Source: CAD feature listing. Evaluate the final solid. Frame: model axes, mm. Face numbers are marked on the shaded views. A direction names the side the tool comes from. Coordinates: 2 decimals unless noted, no trailing zeros. Loops run counter-clockwise (first coordinate to the right, second up) from the corner with the lowest first, then second, coordinate; pieces in that order, holes last. Notation, with made-up numbers: (78.25, 5) -> (101.25, 5) arc R23 ccw to (101.25, 40) -> close; hole circle Ø1 at (-28, 48.5). An arc over 180 degrees is marked (long way). Answer as CSV lines item,"result".
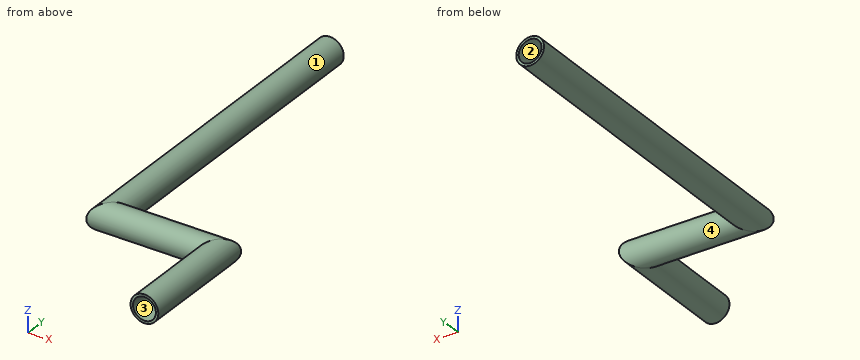
from build123d import *

# Parameters (mm, degrees)
SKETCH2_R   = 12.7
SKETCH2_R_2 = 10.458255758


with BuildPart() as part:
    # Sweep1: sweep along a path in Sketch1
    with BuildLine(Plane.XY) as sweep1_path:
        Line((0, 300), (0, 0))
        Line((0, 0), (99.24397827, 0))
        Line((99.24397827, 0), (99.24397827, -100))
    # Sketch2 → Sweep1 (sweep)
    with BuildSketch(Plane(origin=(0, 300, 0), x_dir=(1, 0, 0), z_dir=(0, 1, 0))):
        Circle(SKETCH2_R)
        Circle(SKETCH2_R_2, mode=Mode.SUBTRACT)
    sweep(path=sweep1_path.line, transition=Transition.RIGHT)


solid = part.part
(1) Cut plane D-D (x = 83). Return the cut outline in (y, z).
Computed values:
outline,"circle Ø25.4 at (0, 0); hole circle Ø20.92 at (0, 0)"
(2) Pin query (flat end, axial travel): pin 1 Ø5 at (x, y) = (4.5, 231) entering from -Z; pin 2 Ø6 at (x, z) = (63.5, 8) entering from -Y; pin 3 Ø12.5 at (x, z) = (0, 0) entering from +Y. Return the tip coordinate at first contact, or that it passes through.
Computed values:
pin 1,"z = -12.54"
pin 2,"y = -11.67"
pin 3,"y = -8.39"
(3) Cut plane B-B (x = 0). Return the cut outline in (y, z), then the cut area to 3 significant figures.
Computed values:
outline,"(0, -12.7) -> (300, -12.7) -> (300, -10.46) -> (0, -10.46) arc R10.46 cw to (0, 10.46) -> (300, 10.46) -> (300, 12.7) -> (0, 12.7) arc R12.7 ccw to start"
area,"1,430 mm^2"
(4) Draft query along Z for the marked faces 1 and 2. Return one class per face: released by +Z, released by -Z, zero draft, split by the parting line, or undercut.
Computed values:
face 1,"split by the parting line"
face 2,"undercut"
(5) Cut plane C-C (y = 0). Return the cut outline in (x, z), then the cut area to 3 significant figures.
Computed values:
outline,"(0, -12.7) -> (99.24, -12.7) arc R12.7 ccw to (99.24, 12.7) -> (0, 12.7) arc R12.7 ccw to start; hole (0, -10.46) -> (99.24, -10.46) arc R10.46 ccw to (99.24, 10.46) -> (0, 10.46) arc R10.46 ccw to start"
area,"608 mm^2"
(6) Material intervals for L1, parallel to X at y = -38, z = 0; L2, parallel to Z at x = 0, y = 233, sorted ascending. Write a range as [from, to].
Computed values:
L1,"[86.54, 88.79], [109.7, 111.94]"
L2,"[-12.7, -10.46], [10.46, 12.7]"
(7) Cut plane A-A (z = 0). Return the cut outline in (x, y).
Computed values:
outline,"(-12.7, -12.7) -> (86.54, -12.7) -> (86.54, -100) -> (88.79, -100) -> (88.79, -10.46) -> (-10.46, -10.46) -> (-10.46, 300) -> (-12.7, 300) -> close; (10.46, 10.46) -> (109.7, 10.46) -> (109.7, -100) -> (111.94, -100) -> (111.94, 12.7) -> (12.7, 12.7) -> (12.7, 300) -> (10.46, 300) -> close"
(8) Access query for the marked faces 3 and 4. Directions: +Z, -Z, +X, -X, +Y, -Y. A direction counts if a zero-diameter tool reaches every point of the face in a straight line with its end or side. Return the directions, or none.
Computed values:
face 3,"-Y"
face 4,"none"
